Geometry: see drawing. Coordinates: mm, zero at the bounding-box minimum. A direction names the side the tool comes from. Coordinates: 2 decimals unless noted, no trailing zeros. Loops run counter-clockwise (first coordinate to the right, second up) from the corner with the lowest first, then second, coordinate; pieces in that order, holes last.
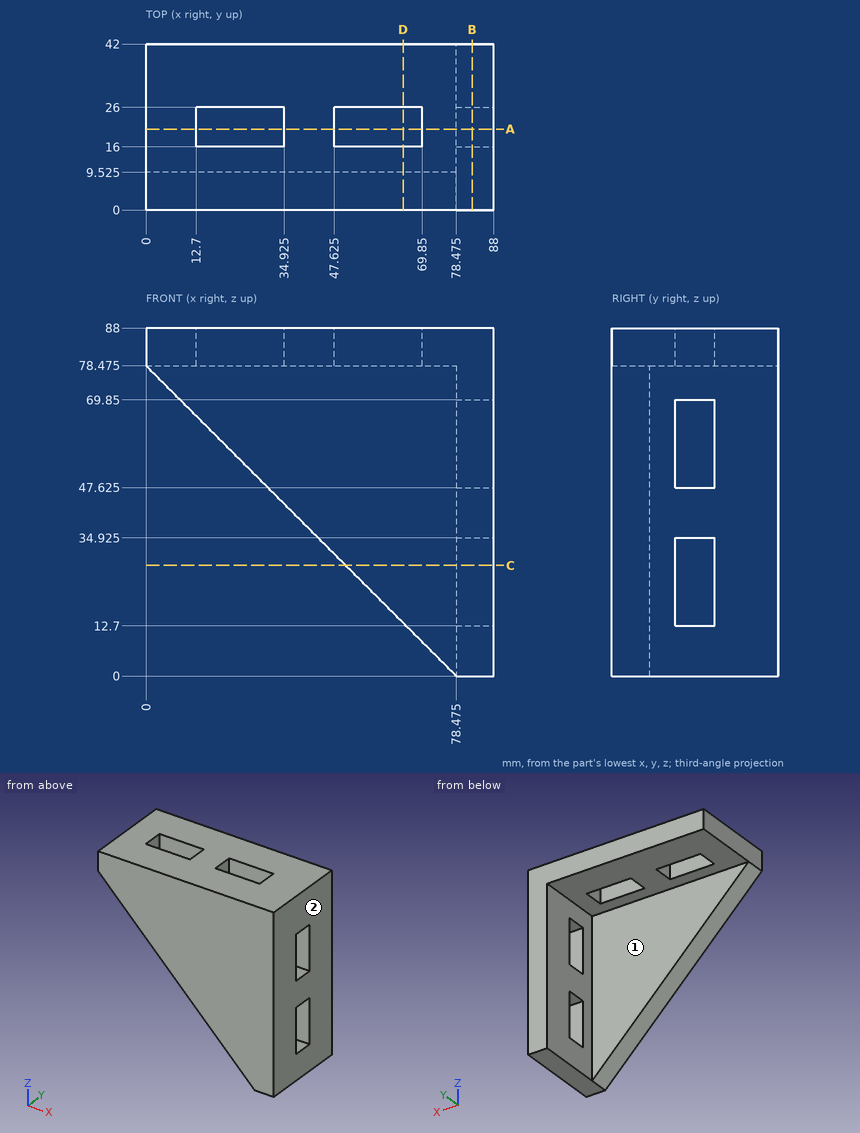
Item 1: Reachability of the marked faces 1 and 2 from +Z, -Z, +X, -X, +Y, -Y: full face, straight path, thin tool, end or side. Return the list, or none.
Result:
face 1: -Z, -X, +Y
face 2: +Z, -Z, +X, +Y, -Y
Item 2: Contact query for flat-ended pins moving along their axis: P1, Ø1.5, axis at x = 74.5, z = 24.5, coming from the -Y side; P2, Ø16, axis at x = 43, y = 30.5, coming from the -Z side (3 decimals); P3, Ø8, axis at x = 58, z = 32, coming from the +Y side (3 decimals). Output: stop coordinate, or through.
Result:
P1: stops at y = 0
P2: stops at z = 78.475
P3: stops at y = 9.525
Item 3: Section query D-D (x = 65). Output: boundary loops of the cut face in (y, z) (3 decimals), then the cut area to 3 significant figures.
Result:
outline: (0, 13.475) - (9.525, 13.475) - (9.525, 78.475) - (16, 78.475) - (16, 88) - (0, 88) - close; (26, 78.475) - (42, 78.475) - (42, 88) - (26, 88) - close
area: 924 mm2
Item 4: Section query C-C (z = 28). Output: boundary loops of the cut face in (x, y) (3 decimals), then the cut area to 4 significant figures.
Result:
outline: (50.475, 0) - (88, 0) - (88, 16) - (78.475, 16) - (78.475, 9.525) - (50.475, 9.525) - close; (78.475, 26) - (88, 26) - (88, 42) - (78.475, 42) - close
area: 571.5 mm2
Item 5: Section query A-A (y = 20.5). Output: boundary loops of the cut face in (x, z) (3 decimals).
Result:
outline: (0, 78.475) - (12.7, 78.475) - (12.7, 88) - (0, 88) - close; (34.925, 78.475) - (47.625, 78.475) - (47.625, 88) - (34.925, 88) - close; (69.85, 78.475) - (78.475, 78.475) - (78.475, 69.85) - (88, 69.85) - (88, 88) - (69.85, 88) - close; (78.475, 0) - (88, 0) - (88, 12.7) - (78.475, 12.7) - close; (78.475, 34.925) - (88, 34.925) - (88, 47.625) - (78.475, 47.625) - close
Item 6: Section query B-B (x = 82.5). Output: boundary loops of the cut face in (y, z) (3 decimals).
Result:
outline: (0, 0) - (42, 0) - (42, 88) - (0, 88) - close; hole (16, 12.7) - (26, 12.7) - (26, 34.925) - (16, 34.925) - close; hole (16, 47.625) - (26, 47.625) - (26, 69.85) - (16, 69.85) - close
Item 7: Line query: L1, parallel to X at y = 23.5, z = 79.5 (3 decimals); L2, parallel to Y at x = 58.5, z = 82. Output: solid intervals per line, ascending.
Result:
L1: x = 0 to 12.7, 34.925 to 47.625, 69.85 to 88
L2: y = 0 to 16, 26 to 42
